```python
from build123d import *

# Parameters (mm, degrees)
SKETCH1_W           = 60
SKETCH1_H           = 60
BOSS_EXTRUDE1_DEPTH = 13
SKETCH2_W           = 15
SKETCH2_H           = 60
BOSS_EXTRUDE2_DEPTH = 8
SKETCH3_R           = 1.15
CUT_EXTRUDE1_DEPTH  = 48.339201514
SKETCH4_R           = 2.2
CUT_EXTRUDE2_DEPTH  = 18
CUT_EXTRUDE4_DEPTH  = 71.292247083


with BuildPart() as part:
    # Sketch1 → Boss-Extrude1 (new body)
    with BuildSketch(Plane.XY):
        Rectangle(SKETCH1_W, SKETCH1_H)
    extrude(amount=BOSS_EXTRUDE1_DEPTH)

    # Sketch2 → Boss-Extrude2 (add)
    with BuildSketch(Plane.XY.offset(13)):
        with Locations((-22.5, 0)):
            Rectangle(SKETCH2_W, SKETCH2_H)
        with Locations((22.5, 0)):
            Rectangle(SKETCH2_W, SKETCH2_H)
    extrude(amount=BOSS_EXTRUDE2_DEPTH)

    # Sketch3 → Cut-Extrude1 (cut, through all)
    with BuildSketch(Plane(origin=(0, 0, 0), x_dir=(-1, 0, 0), z_dir=(0, 0, -1))):
        with Locations((25, 25)):
            Circle(SKETCH3_R)
        with Locations((25, -25)):
            Circle(SKETCH3_R)
        with Locations((-25, -25)):
            Circle(SKETCH3_R)
        with BuildLine():
            ThreePointArc((-25.813172798, 25.813172798), (-25.813172798, 24.186827202), (-24.186827202, 24.186827202))
            Line((-24.186827202, 24.186827202), (-25.813172798, 25.813172798))
        make_face()
        with BuildLine():
            Line((-25.813172798, 25.813172798), (-24.186827202, 24.186827202))
            ThreePointArc((-24.186827202, 24.186827202), (-23.937538538, 24.559914053), (-23.85, 25))
            ThreePointArc((-23.85, 25), (-24.559914053, 26.062461462), (-25.813172798, 25.813172798))
        make_face()
    extrude(amount=-CUT_EXTRUDE1_DEPTH, mode=Mode.SUBTRACT)

    # Sketch4 → Cut-Extrude2 (cut)
    with BuildSketch(Plane(origin=(0, 0, 0), x_dir=(-1, 0, 0), z_dir=(0, 0, -1))):
        with Locations((-25, 25)):
            Circle(SKETCH4_R)
        with Locations((25, 25)):
            Circle(SKETCH4_R)
        with Locations((25, -25)):
            Circle(SKETCH4_R)
        with Locations((-25, -25)):
            Circle(SKETCH4_R)
    extrude(amount=-CUT_EXTRUDE2_DEPTH, mode=Mode.SUBTRACT)

    # Sketch6 → Cut-Extrude4 (cut, through all)
    with BuildSketch(Plane(origin=(0, 30, 0), x_dir=(1, 0, 0), z_dir=(0, 1, 0))):
        Polygon((-30, 0), (-30, -13), (-20, -13), (-13.5, 0), align=None)
        Polygon((30, 0), (13.5, 0), (20, -13), (30, -13), align=None)
    extrude(amount=-CUT_EXTRUDE4_DEPTH, mode=Mode.SUBTRACT)


solid = part.part
```
CAD build for the part. Positions are in the model's coordinates, mm. A direction names the side the tool comes from. Coordinates: 2 decimals unless noted, no trailing zeros. Order: outer loops, then holes, each group sorted by start corner. A loop starts at its lowest first (then second) coordinate and runs counter-clockwise, first axis right, second up. Notation, with made-up numbers: M 74,54 L 109,54 A25 ccw 109,90 Z; hole C 49.5,-18 d8. An arc over 180 degrees is marked long. Write each question's results on one line, items separated by ' | '. Start each with the question number.
Q1. Flat gauge pins, fed straight in: P1, Ø6, axis at y = -6, z = 4.5, coming from the +X side; P2, Ø11, axis at x = -23, y = -9.5, coming from the -Z side; P3, Ø1.5, axis at x = -2.5, y = 19.5, coming from the +Z side; P4, Ø1.8, axis at x = -25, y = -25, coming from the -Z side. Where does each tip first touch, or does it go through?
Q2. Pull direction Y, two halves, no side cores. Call faces 1 (the cylindrical face through (-24.751, -26.123, 19.479)), 2 (the flat face through (22, 0, 21)), 3 (the flat face through (0, 30, 10)): +Y half, -Y half, draft (parallel to the pull), parting line (faces both ways), or undercut.
Q3. Cut at C-C (z = 5.5). List the corners of the cut face in (x, y), then the cut area to 3 significant figures.
Q4. Cut at D-D (x = -3). List the corners of the cut face in (y, z).
Q5. Drill centre lines: probe 1 along Y at (x, z) = (25, 19.6); probe 2 along X at (y, z) = (-16, 16); probe 3 along Y at (x, z) = (25, 16.95). Where is each one in solid material? Low to high. Write a range as from..to.
Q6. Which spindle directions (+Z, -Z, +X, -X, +Y, -Y) get a long thin tool onto all of the face, cutting with end or side? Do faces 4 (the flat face through (-25, 0, 13)), 5 (the cylindrical face through (25.477, -27.148, 15.465)), 6 (the flat face through (25, 0, 13)), 7 (the flat face through (0, 0, 13)). Say none if no direction does.
Q7. Cut at B-B (y = 14). List the corners of the cut face in (x, z).
Q8. Cut at A-A (x = 25). List the corners of the cut face in (y, z), then the cut area to 3 significant figures.
Found:
1) P1: x = 17.25 | P2: z = 8 | P3: z = 13 | P4: through
2) face 1: undercut | face 2: draft | face 3: +Y half
3) outline: M -16.25,-30 L 16.25,-30 L 16.25,30 L -16.25,30 Z | area: 1,950 mm²
4) outline: M -30,0 L 30,0 L 30,13 L -30,13 Z
5) probe 1: -30..-26.15, -23.85..23.85, 26.15..30 | probe 2: -30..-15, 15..30 | probe 3: -30..-27.2, -22.8..22.8, 27.2..30
6) face 4: -Z, -X, +Y, -Y | face 5: -Z | face 6: -Z, +X, +Y, -Y | face 7: +Z, +Y, -Y
7) outline: M -30,13 L -20,13 L -13.5,0 L 13.5,0 L 20,13 L 30,13 L 30,21 L 15,21 L 15,13 L -15,13 L -15,21 L -30,21 Z
8) outline: M -30,13 L -27.2,13 L -27.2,18 L -26.15,18 L -26.15,21 L -30,21 Z; M -23.85,18 L -22.8,18 L -22.8,13 L 22.8,13 L 22.8,18 L 23.85,18 L 23.85,21 L -23.85,21 Z; M 26.15,18 L 27.2,18 L 27.2,13 L 30,13 L 30,21 L 26.15,21 Z | area: 422 mm²
